```python
from build123d import *

# Parameters (mm, degrees)
BOSS_EXTRUDE1_DEPTH = 25
CUT_EXTRUDE2_DEPTH  = 20
SKETCH6_R           = 3
CUT_EXTRUDE5_DEPTH  = 400
BOSS_EXTRUDE2_DEPTH = 5
SKETCH8_R           = 3
CUT_EXTRUDE6_DEPTH  = 350
FILLET3_R           = 2
SKETCH9_R           = 4
CUT_EXTRUDE7_DEPTH  = 350


with BuildPart() as part:
    # Sketch1 → Boss-Extrude1 (new body)
    with BuildSketch(Plane.XY):
        Polygon((0, 0), (0, 180), (300, 180), (300, 0), (270, 0), (270, 150), (30, 150), (30, 0), align=None)
    extrude(amount=BOSS_EXTRUDE1_DEPTH)

    # Sketch3 → Cut-Extrude2 (cut)
    with BuildSketch(Plane(origin=(0, 0, 0), x_dir=(-1, 0, 0), z_dir=(0, 0, -1))):
        Polygon((-5, 0), (-30, 0), (-30, 150), (-270, 150), (-270, 0), (-295, 0), (-295, 175), (-5, 175), align=None)
    extrude(amount=-CUT_EXTRUDE2_DEPTH, mode=Mode.SUBTRACT)

    # Sketch6 → Cut-Extrude5 (cut)
    with BuildSketch(Plane.XY.offset(25)):
        with Locations((15, 30)):
            Circle(SKETCH6_R)
        with Locations((285, 30)):
            Circle(SKETCH6_R)
    extrude(amount=-CUT_EXTRUDE5_DEPTH, mode=Mode.SUBTRACT)

    # Sketch7 → Boss-Extrude2 (add)
    with BuildSketch(Plane(origin=(0, 0, 0), x_dir=(-1, 0, 0), z_dir=(0, 0, -1))):
        Polygon((-300, 0), (-300, 180), (0, 180), (0, 0), (-5, 0), (-5, 175), (-295, 175), (-295, 0), align=None)
    extrude(amount=BOSS_EXTRUDE2_DEPTH)

    # Sketch8 → Cut-Extrude6 (cut)
    with BuildSketch(Plane.ZY):
        with Locations((10, 30)):
            Circle(SKETCH8_R)
    extrude(amount=-CUT_EXTRUDE6_DEPTH, mode=Mode.SUBTRACT)

    # Fillet3
    fillet3_edges = [part.edges().sort_by_distance(p)[0] for p in [
        (270, 150, 22.5),
        (30, 150, 22.5),
        (5, 87.5, 20),
        (5, 175, 7.5),
        (295, 87.5, 20),
        (150, 175, 20),
        (295, 175, 7.5),
    ]]
    fillet(fillet3_edges, radius=FILLET3_R)

    # Sketch9 → Cut-Extrude7 (cut)
    with BuildSketch(Plane(origin=(0, 180, 0), x_dir=(1, 0, 0), z_dir=(0, 1, 0))):
        with Locations(Location((40, -10, 0), (0, 0, 270))):
            Circle(SKETCH9_R)
        with Locations(Location((260, -10, 0), (0, 0, 270))):
            Circle(SKETCH9_R)
    extrude(amount=-CUT_EXTRUDE7_DEPTH, mode=Mode.SUBTRACT)


solid = part.part
```
Model file for the job. Use its own axes, mm. A direction names the side the tool comes from. Round coordinates to 2 decimals unless told otherwise and drop trailing zeros. Order: outer loops, then holes, each group sorted by start corner. A loop starts at its lowest first (then second) coordinate and runs counter-clockwise, first axis right, second up. Notation, with made-up numbers: M 3.25,-8 L 58.25,-8 A18 ccw 58.25,2 Z; hole C 27,-39 d8. An arc over 180 degrees is marked long. Use CSV: the item, a comma, the result in double quotes.
Item 1: Pull direction Y, two halves, no side cores. Call faces 3 (the face through (295, 88, 7)), 4 (the face through (148, 175, 7)), 5 (the face through (282, 30, 23)): released by +Y, released by -Y, zero draft, split by the parting line, or undercut.
Worked answers:
face 3,"zero draft"
face 4,"released by -Y"
face 5,"undercut"
Item 2: Saw through at C-C (y = 138). List the corners of the cut face in (x, z).
Worked answers:
outline,"M 0,-5 L 5,-5 L 5,18 A2 cw 7,20 L 30,20 L 30,25 L 0,25 Z; M 270,20 L 293,20 A2 cw 295,18 L 295,-5 L 300,-5 L 300,25 L 270,25 Z"
Item 3: Probe probe 1 along X at (y, z) = (177.45, 10); probe 2 along X at (y, z) = (119.5, 5); probe 3 along Z at (x, y) = (260, 176.1). List the from-to ranges inside material, lowest first.
Worked answers:
probe 1,"0 to 36, 44 to 256, 264 to 300"
probe 2,"0 to 5, 295 to 300"
probe 3,"-5 to 6, 14 to 25"
Item 4: Saw through at A-A (z = 10). List the corners of the cut face in (x, y).
Worked answers:
outline,"M 0,0 L 5,0 L 5,27 L 0,27 Z; M 0,33 L 5,33 L 5,173 A2 cw 7,175 L 36,175 L 36,180 L 0,180 Z; M 44,175 L 256,175 L 256,180 L 44,180 Z; M 264,175 L 293,175 A2 cw 295,173 L 295,33 L 300,33 L 300,180 L 264,180 Z; M 295,0 L 300,0 L 300,27 L 295,27 Z"
Item 5: Saw through at D-D (y = 30). State how many separate pieces and enclosed holes the cut face has, plus the area to 3 significant figures.
Worked answers:
separate pieces,"6"
enclosed holes,"0"
area,"432 mm²"
Item 6: Saw through at B-B (x = 15). List the corners of the cut face in (y, z).
Worked answers:
outline,"M 0,20 L 27,20 L 27,25 L 0,25 Z; M 33,20 L 173,20 A2 cw 175,18 L 175,-5 L 180,-5 L 180,25 L 33,25 Z"
Item 7: Which spindle directions (+Z, -Z, +X, -X, +Y, -Y) get a long thin tool onto all of the face, cutting with end or side? Do faces 1 (the face through (297.46, 28.85, 12.77)), 2 (the face through (5, 85, 7)). Say none if no direction does.
Worked answers:
face 1,"+X, -X"
face 2,"-Z, -Y"
Item 8: Pin check, flat tips, straight feed: pin 1 (5 mm diameter, centred on x = 48, y = 148, fed in from -Z); pin 2 (10.5 mm diameter, centred on x = 260, z = 10, fed in from -Y); pin 3 (2.5 mm diameter, centred on x = 158, z = 23.5, fed in from -Y). Stop position of each tip, or through.
Worked answers:
pin 1,"z = 20"
pin 2,"y = 175"
pin 3,"y = 150"
